from build123d import *

# Parameters (mm, degrees)
SKETCH1_W           = 60
SKETCH1_H           = 8
BOSS_EXTRUDE1_DEPTH = 20
CUT_EXTRUDE1_DEPTH  = 64.749509802
SKETCH4_R           = 1.5
CUT_EXTRUDE2_DEPTH  = 64.749509802


with BuildPart() as part:
    # Sketch1 → Boss-Extrude1 (new body)
    with BuildSketch(Plane.XY):
        with Locations((30, -4)):
            Rectangle(SKETCH1_W, SKETCH1_H)
    extrude(amount=BOSS_EXTRUDE1_DEPTH)

    # Sketch2 → Cut-Extrude1 (cut, through all)
    with BuildSketch(Plane(origin=(60, 0, 0), x_dir=(0, 0, -1), z_dir=(1, 0, 0))):
        Polygon((0, -4), (0, -2.5), (-3, -2.5), (-3, -0.7), (-10, -0.7), (-10, -7.3), (-3, -7.3), (-3, -5.5), (0, -5.5), align=None)
    extrude(amount=-CUT_EXTRUDE1_DEPTH, mode=Mode.SUBTRACT)

    # Sketch4 → Cut-Extrude2 (cut, through all)
    with BuildSketch(Plane(origin=(0, 0, 0), x_dir=(1, 0, 0), z_dir=(0, 1, 0))):
        with Locations(Location((40, -15, 0), (0, 0, 270))):
            Circle(SKETCH4_R)
        with Locations(Location((20, -15, 0), (0, 0, 270))):
            Circle(SKETCH4_R)
    extrude(amount=-CUT_EXTRUDE2_DEPTH, mode=Mode.SUBTRACT)


solid = part.part
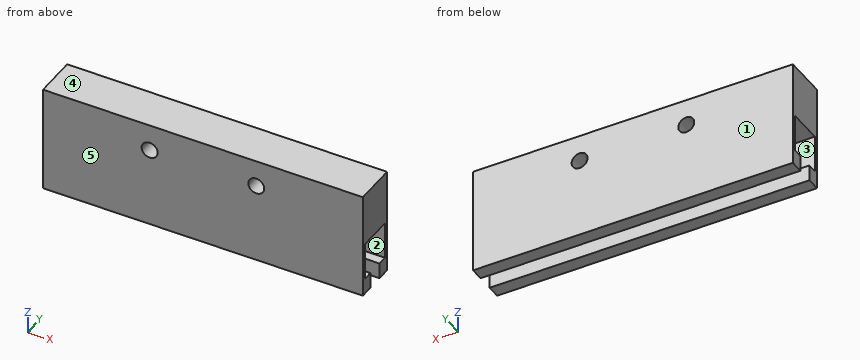
CAD build for the part. Positions are in the model's coordinates, mm. Face numbers are marked on the shaded views. A direction names the side the tool comes from. Round coordinates to 2 decimals unless told otherwise and drop trailing zeros. Write each loop counter-clockwise with the first axis right and the second up, starting at its lowest first coordinate (ties: lowest second). Pieces come first, ordered by that corner, then holes. Notation, with made-up numbers: M -39.75,-14 L -18.75,-14 A15 cw -18.75,2 Z; hole C 78,-21.75 d1. An arc over 180 degrees is marked long. Put each result on its own line as item: value. Start each with the question number.
1) Pin check, flat tip, straight feed: pin 1 Ø2.5 at (x, z) = (40, 15) entering from +Y. Stop position of the tip, or through.
2) 3-axis set-ups, long thin cutter, end or side, ignore diameter. For the marked faces 1 and 2: which of +Z, -Z, +X, -X, +Y, -Y reach the whole face in a straight line?
3) Drill centre lines: probe 1 along X at (y, z) = (-5.5, 15); probe 2 along Z at (x, y) = (34, -7.25); probe 3 along Y at (x, z) = (41.5, 8.5). Where is each one in solid material? Low to high. Write a range as [from, to].
4) Saw through at D-D, the plane z = 15. Write the cut outline in (x, y), and give its area (3 significant figures).
5) Saw through at C-C, the plane x = 55.5. Write the cut outline in (y, z).
6) Saw through at A-A, the plane y = -6.75. Write the cut outline in (x, z), and give its area (3 significant figures).
7) Saw through at B-B, the plane z = 1.75. Write the cut outline in (x, y), and give its area (3 significant figures).
8) Pull direction Y, two halves, no side cores. Call the marked faces 3, 4 and 5: pulls with the +Y half, pulls with the -Y half, needs draft (parallel to the pull), parting line crosses it, or undercut.
Resolved:
1. pin 1: through
2. face 1: +Z, -Z, +X, -X, +Y
2. face 2: +X, -X
3. probe 1: [0, 18.5], [21.5, 38.5], [41.5, 60]
3. probe 2: [0, 3], [10, 20]
3. probe 3: [-8, -7.3], [-0.7, 0]
4. outline: M 0,-8 L 18.5,-8 L 18.5,0 L 0,0 Z; M 21.5,-8 L 38.5,-8 L 38.5,0 L 21.5,0 Z; M 41.5,-8 L 60,-8 L 60,0 L 41.5,0 Z
4. area: 432 mm²
5. outline: M -8,0 L -5.5,0 L -5.5,3 L -7.3,3 L -7.3,10 L -0.7,10 L -0.7,3 L -2.5,3 L -2.5,0 L 0,0 L 0,20 L -8,20 Z
6. outline: M 0,0 L 60,0 L 60,3 L 0,3 Z; M 0,10 L 60,10 L 60,20 L 0,20 Z; hole C 20,15 d3; hole C 40,15 d3
6. area: 766 mm²
7. outline: M 0,-8 L 60,-8 L 60,-5.5 L 0,-5.5 Z; M 0,-2.5 L 60,-2.5 L 60,0 L 0,0 Z
7. area: 300 mm²
8. face 3: undercut
8. face 4: needs draft
8. face 5: pulls with the -Y half
